Can you work these out from the model? Positions are in its coordinate system, mm. A direction names the side the tool comes from. Give positions to 0.01 mm unless a question says otherwise; leave off trailing zeros. Order: outer loops, then holes, each group sorted by start corner. A loop starts at its lowest first (then second) coordinate and runs counter-clockwise, first axis right, second up.
Item 1: I want a section at D-D, the plane z = 2.5. Write out the boundary of the cut face in (x, y), then the cut area to 3 significant figures.
Item 2: I'm going to push a flat-ended pin straight in: pin 1 Ø3.5 at (x, y) = (6.5, 3) entering from +Z. Where does the tip first touch, or does it pass through?
Item 3: If I drill on line 1 along X through (y, z) = (3.5, 5); line 2 along X through (y, z) = (0.5, 1); line 3 along Z through (x, y) = (17.9, -3), over which ranges is the centre line in solid material (lowest first)?
Item 4: Which directions (+Z, -Z, +X, -X, +Y, -Y) give clear straight access to the entire face, cutting with the end or side of a thin tool? Please do faces 1 (the cylindrical face through (-17.986, 2.675, 5.536)), 2 (the cylindrical face through (0, 3.7, 0.8)), 3 (the flat face through (-17, 0, 5)).
Item 5: If we mould it in two halves opening along Y, with no side actions, what happens to faces 4 (the flat face through (-2.2, 0, 1)), 5 (the cylindrical face through (-17.99, -5.1, 8.64)), 6 (the flat face through (0, 4, 0)), 7 (the cylindrical face through (-17.99, -2.31, 5.67))? For each: +Y half, -Y half, draft (parallel to the pull), parting line (faces both ways), or undercut.
Item 6: I want a section at C-C, the plane y = 1. Write out the boundary of the cut face in (x, z).
Item 7: I want a section at B-B, the plane z = 1. Write out the boundary of the cut face in (x, y), then the cut area to 3 significant figures.
Item 8: I want a section at A-A, the plane x = 0. Write out the boundary of the cut face in (y, z).
```python
from build123d import *

# Parameters (mm, degrees)
SKETCH1_W      = 38
SKETCH1_H      = 12
EXTRUDE1_DEPTH = 1.5
SKETCH2_W      = 2
SKETCH2_H      = 12
EXTRUDE2_DEPTH = 8
EXTRUDE3_REACH = 41.626
SKETCH3_R      = 1.5
FILLET1_R      = 3
EXTRUDE4_DEPTH = 1.5


with BuildPart() as part:
    # Sketch1 → Extrude1 (new body)
    with BuildSketch(Plane.XY):
        Rectangle(SKETCH1_W, SKETCH1_H)
    extrude(amount=EXTRUDE1_DEPTH)

    # Sketch2 → Extrude2 (add)
    with BuildSketch(Plane.XY.offset(1.5)):
        with Locations((-18, 0)):
            Rectangle(SKETCH2_W, SKETCH2_H)
        with Locations((18, 0)):
            Rectangle(SKETCH2_W, SKETCH2_H)
    extrude(amount=EXTRUDE2_DEPTH)

    # Extrude3: up to this face of the body (flat: up to its plane)
    extrude3_end = Plane(part.part.faces().sort_by_distance((-19, 0, 4.75))[0])
    # Sketch3 → Extrude3 (cut, up to the picked face)
    with BuildSketch(Plane(origin=(19, 0, 0), x_dir=(0, 0, -1), z_dir=(1, 0, 0)), mode=Mode.PRIVATE) as extrude3_sk1:
        with Locations(Location((-7, 3, 0), (0, 0, 90))):
            Circle(SKETCH3_R)
    extrude3_tool1 = split(extrude(extrude3_sk1.sketch, amount=-EXTRUDE3_REACH, mode=Mode.PRIVATE), bisect_by=extrude3_end, keep=Keep.BOTH, mode=Mode.PRIVATE)
    # Sketch3 → Extrude3 (cut, up to the picked face)
    with BuildSketch(Plane(origin=(19, 0, 0), x_dir=(0, 0, -1), z_dir=(1, 0, 0)), mode=Mode.PRIVATE) as extrude3_sk2:
        with Locations(Location((-7, -3, 0), (0, 0, 90))):
            Circle(SKETCH3_R)
    extrude3_tool2 = split(extrude(extrude3_sk2.sketch, amount=-EXTRUDE3_REACH, mode=Mode.PRIVATE), bisect_by=extrude3_end, keep=Keep.BOTH, mode=Mode.PRIVATE)
    add(extrude3_tool1.solids().sort_by(Axis((19, 3, 7), (-1, 0, 0)))[0], mode=Mode.SUBTRACT)
    add(extrude3_tool2.solids().sort_by(Axis((19, -3, 7), (-1, 0, 0)))[0], mode=Mode.SUBTRACT)

    # Fillet1
    fillet1_edges = [part.edges().sort_by_distance(p)[0] for p in [
        (18, 6, 9.5),
        (18, -6, 9.5),
        (-18, -6, 9.5),
        (-18, 6, 9.5),
    ]]
    fillet(fillet1_edges, radius=FILLET1_R)

    # Sketch4 → Extrude4 (cut)
    with BuildSketch(Plane.XY.offset(1.5)):
        with BuildLine():
            Line((-2.2, 1.5), (-2.2, -1.5))
            ThreePointArc((-2.2, -1.5), (0, -3.7), (2.2, -1.5))
            Line((2.2, -1.5), (2.2, 1.5))
            ThreePointArc((2.2, 1.5), (0, 3.7), (-2.2, 1.5))
        make_face()
    extrude(amount=-EXTRUDE4_DEPTH, mode=Mode.SUBTRACT)


solid = part.part
```
Results list:
1. outline: (-19, -6) - (-17, -6) - (-17, 6) - (-19, 6) - close; (17, -6) - (19, -6) - (19, 6) - (17, 6) - close
1. area: 48.0 mm2
2. pin 1: stops at z = 1.5
3. line 1: x = -19 to -17, 17 to 19
3. line 2: x = -19 to -2.2, 2.2 to 19
3. line 3: z = 0 to 5.5, 8.5 to 9.5
4. face 1: +X, -X
4. face 2: +Z, -Z
4. face 3: +Z, +Y, -Y
5. face 4: undercut
5. face 5: -Y half
5. face 6: draft
5. face 7: undercut
6. outline: (-19, 0) - (-2.2, 0) - (-2.2, 1.5) - (-17, 1.5) - (-17, 9.5) - (-19, 9.5) - close; (2.2, 0) - (19, 0) - (19, 9.5) - (17, 9.5) - (17, 1.5) - (2.2, 1.5) - close
7. outline: (-19, -6) - (19, -6) - (19, 6) - (-19, 6) - close; hole (-2.2, -1.5) arc R2.2 ccw to (2.2, -1.5) - (2.2, 1.5) arc R2.2 ccw to (-2.2, 1.5) - close
7. area: 428 mm2
8. outline: (-6, 0) - (-3.7, 0) - (-3.7, 1.5) - (-6, 1.5) - close; (3.7, 0) - (6, 0) - (6, 1.5) - (3.7, 1.5) - close
